Design review of the part built by this model. Coordinates are the model's own, in mm. Give positions to 0.01 mm unless a question says otherwise; leave off trailing zeros. Write each loop counter-clockwise with the first axis right and the second up, starting at its lowest first coordinate (ties: lowest second). Pieces come first, ordered by that corner, then holes.
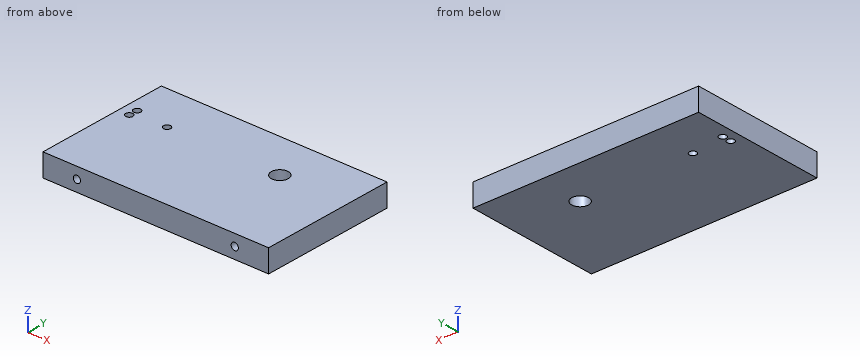
```python
from build123d import *

# Parameters (mm, degrees)
SKETCH1_W                       = 127
SKETCH1_H                       = 76.2
BOSS_EXTRUDE1_DEPTH             = 12.7
F_1_32_0_159_DIAMETER_HOLE1_D   = 4.0386
F_10_32_TAPPED_HOLE1_D          = 4.0386
F_10_32_TAPPED_HOLE1_DEPTH      = 11.486682152
F_10_32_TAPPED_HOLE1_TIP        = 1.213317848
F_3_8_0_375_DIAMETER_HOLE1_D    = 9.525
F_10_32_TAPPED_HOLE2_D          = 4.0386
F_10_32_TAPPED_HOLE2_DEPTH      = 14.478
F_10_32_TAPPED_HOLE2_TIP        = 1.213317848
F_21_0_159_DIAMETER_HOLE1_D     = 4.0386
F_21_0_159_DIAMETER_HOLE1_DEPTH = 14.478
F_21_0_159_DIAMETER_HOLE1_TIP   = 1.213317848


with BuildPart() as part:
    # Sketch1 → Boss-Extrude1 (new body)
    with BuildSketch(Plane.XY):
        with Locations((63.5, 38.1)):
            Rectangle(SKETCH1_W, SKETCH1_H)
    extrude(amount=BOSS_EXTRUDE1_DEPTH)

    # 1/32 (0.159) Diameter Hole1 (through all)
    with Locations(Plane.XY.offset(12.7)):
        with Locations((25.4, 50.8)):
            Hole(F_1_32_0_159_DIAMETER_HOLE1_D / 2)

    # #10-32 Tapped Hole1
    with Locations(Plane(origin=(0, 0, 0), x_dir=(-1, 0, 0), z_dir=(0, -1, 0))):
        with Locations((-19.05, -6.35), (-107.95, -6.35)):
            Hole(F_10_32_TAPPED_HOLE1_D / 2, depth=F_10_32_TAPPED_HOLE1_DEPTH)
            with Locations((0, 0, -(F_10_32_TAPPED_HOLE1_DEPTH + F_10_32_TAPPED_HOLE1_TIP / 2))):  # 118° drill point
                Cone(0, F_10_32_TAPPED_HOLE1_D / 2, F_10_32_TAPPED_HOLE1_TIP, mode=Mode.SUBTRACT)

    # 3/8 (0.375) Diameter Hole1 (through all)
    with Locations(Plane.XY.offset(12.7)):
        with Locations((88.9, 50.8)):
            Hole(F_3_8_0_375_DIAMETER_HOLE1_D / 2)

    # #10-32 Tapped Hole2
    with Locations(Plane.XY.offset(12.7)):
        with Locations((6.35, 48.26)):
            Hole(F_10_32_TAPPED_HOLE2_D / 2, depth=F_10_32_TAPPED_HOLE2_DEPTH)
            with Locations((0, 0, -(F_10_32_TAPPED_HOLE2_DEPTH + F_10_32_TAPPED_HOLE2_TIP / 2))):  # 118° drill point
                Cone(0, F_10_32_TAPPED_HOLE2_D / 2, F_10_32_TAPPED_HOLE2_TIP, mode=Mode.SUBTRACT)

    # #21 (0.159) Diameter Hole1
    with Locations(Plane.XY.offset(12.7)):
        with Locations((6.35, 53.34)):
            Hole(F_21_0_159_DIAMETER_HOLE1_D / 2, depth=F_21_0_159_DIAMETER_HOLE1_DEPTH)
            with Locations((0, 0, -(F_21_0_159_DIAMETER_HOLE1_DEPTH + F_21_0_159_DIAMETER_HOLE1_TIP / 2))):  # 118° drill point
                Cone(0, F_21_0_159_DIAMETER_HOLE1_D / 2, F_21_0_159_DIAMETER_HOLE1_TIP, mode=Mode.SUBTRACT)


solid = part.part
```
(1) Consider section B-B, the plane x = 6.35. Give the boundary of the cut face in (y, z), then the cut area to 3 significant figures.
Resolved:
outline: (0, 0) - (46.24, 0) - (46.24, 12.7) - (0, 12.7) - close; (50.28, 0) - (51.32, 0) - (51.32, 12.7) - (50.28, 12.7) - close; (55.36, 0) - (76.2, 0) - (76.2, 12.7) - (55.36, 12.7) - close
area: 865 mm2
(2) To check wall thickness, follow L1, parallel to X at y = 10, z = 6; L2, parallel to Y at x = 25.4, z = 8; L3, parallel to Z at x = 19, y = 7. State the ranges of each line that lie inside material, in increasing order.
Resolved:
L1: x = 0 to 17.06, 21.04 to 105.96, 109.94 to 127
L2: y = 0 to 48.78, 52.82 to 76.2
L3: z = 0 to 4.33, 8.37 to 12.7
(3) Consider section A-A, the plane x = 88.9. Give the boundary of the cut face in (y, z).
Resolved:
outline: (0, 0) - (46.04, 0) - (46.04, 12.7) - (0, 12.7) - close; (55.56, 0) - (76.2, 0) - (76.2, 12.7) - (55.56, 12.7) - close
